```python
from build123d import *

# Parameters (mm, degrees)
BOSS_EXTRUDE1_DEPTH = 58
BOSS_EXTRUDE2_DEPTH = 5
CUT_EXTRUDE1_DEPTH  = 103.78132126
CHAMFER1_SIZE       = 3


with BuildPart() as part:
    # Sketch1 → Boss-Extrude1 (new body)
    with BuildSketch(Plane(origin=(0, 0, 0), x_dir=(1, 0, 0), z_dir=(0, 1, 0))):
        with BuildLine():
            Line((-7, 0), (7, 0))
            ThreePointArc((7, 0), (10.535533906, 1.464466094), (12, 5))
            Line((12, 5), (12, 66.875644347))
            ThreePointArc((12, 66.875644347), (11.829629131, 68.169739573), (11.330127019, 69.375644347))
            Line((11.330127019, 69.375644347), (4.330127019, 81.5))
            ThreePointArc((4.330127019, 81.5), (0, 84), (-4.330127019, 81.5))
            Line((-4.330127019, 81.5), (-11.330127019, 69.375644347))
            ThreePointArc((-11.330127019, 69.375644347), (-11.829629131, 68.169739573), (-12, 66.875644347))
            Line((-12, 66.875644347), (-12, 5))
            ThreePointArc((-12, 5), (-10.535533906, 1.464466094), (-7, 0))
        make_face()
    extrude(amount=BOSS_EXTRUDE1_DEPTH)

    # Sketch2 → Cut-Revolve3 (revolve, cut)
    with BuildSketch(Plane(origin=(0, 0, 0), x_dir=(0, 0, -1), z_dir=(1, 0, 0))):
        Polygon((48, 61), (48, 58), (48, 51.5), (49.5, 50), (48, 48.5), (48, 42), (37.5, 42), (36, 40.5), (34.5, 42), (24, 42), (24, 35.5), (25.5, 34), (24, 32.5), (24, 26), (13.5, 26), (12, 24.5), (10.5, 26), (0, 26), (-2, 26), (-2, 61), align=None)
    revolve(axis=Axis((0, 58, -89), (0, -1, 0)), mode=Mode.SUBTRACT)

    # Sketch3 → Boss-Extrude2 (add)
    with BuildSketch(Plane.XZ):
        with BuildLine():
            Line((-12, -54.599242435), (-12, -57.934874811))
            ThreePointArc((-12, -57.934874811), (0, -55), (12, -57.934874811))
            Line((12, -57.934874811), (12, -54.599242435))
            ThreePointArc((12, -54.599242435), (0, -52), (-12, -54.599242435))
        make_face()
        with BuildLine():
            Line((-12, -62.599242435), (-12, -65.934874811))
            ThreePointArc((-12, -65.934874811), (0, -63), (12, -65.934874811))
            Line((12, -65.934874811), (12, -62.599242435))
            ThreePointArc((12, -62.599242435), (0, -60), (-12, -62.599242435))
        make_face()
        with BuildLine():
            Line((-12, -46.599242435), (-12, -49.934874811))
            ThreePointArc((-12, -49.934874811), (0, -47), (12, -49.934874811))
            Line((12, -49.934874811), (12, -46.599242435))
            ThreePointArc((12, -46.599242435), (0, -44), (-12, -46.599242435))
        make_face()
        with BuildLine():
            Line((-12, -38.599242435), (-12, -41.934874811))
            ThreePointArc((-12, -41.934874811), (0, -39), (12, -41.934874811))
            Line((12, -41.934874811), (12, -38.599242435))
            ThreePointArc((12, -38.599242435), (0, -36), (-12, -38.599242435))
        make_face()
        with BuildLine():
            Line((-12, -30.599242435), (-12, -33.934874811))
            ThreePointArc((-12, -33.934874811), (0, -31), (12, -33.934874811))
            Line((12, -33.934874811), (12, -30.599242435))
            ThreePointArc((12, -30.599242435), (0, -28), (-12, -30.599242435))
        make_face()
        with BuildLine():
            Line((-12, -22.599242435), (-12, -25.934874811))
            ThreePointArc((-12, -25.934874811), (0, -23), (12, -25.934874811))
            Line((12, -25.934874811), (12, -22.599242435))
            ThreePointArc((12, -22.599242435), (0, -20), (-12, -22.599242435))
        make_face()
        with BuildLine():
            Line((-12, -14.599242435), (-12, -17.934874811))
            ThreePointArc((-12, -17.934874811), (0, -15), (12, -17.934874811))
            Line((12, -17.934874811), (12, -14.599242435))
            ThreePointArc((12, -14.599242435), (0, -12), (-12, -14.599242435))
        make_face()
    extrude(amount=BOSS_EXTRUDE2_DEPTH)

    # Sketch4 → Cut-Extrude1 (cut, through all)
    with BuildSketch(Plane.XY):
        with BuildLine():
            Line((12, 16), (8.601411599, 17.071570807))
            ThreePointArc((8.601411599, 17.071570807), (6.817380703, 16.777026114), (6, 15.164136905))
            Line((6, 15.164136905), (6, 8.835863095))
            ThreePointArc((6, 8.835863095), (6.817380703, 7.222973886), (8.601411599, 6.928429193))
            Line((8.601411599, 6.928429193), (12, 8))
            Line((12, 8), (12, 16))
        make_face()
        with BuildLine():
            Line((-12, 8), (-12, 16))
            Line((-12, 16), (-8.601411599, 17.071570807))
            ThreePointArc((-8.601411599, 17.071570807), (-6.817380703, 16.777026114), (-6, 15.164136905))
            Line((-6, 15.164136905), (-6, 8.835863095))
            ThreePointArc((-6, 8.835863095), (-6.817380703, 7.222973886), (-8.601411599, 6.928429193))
            Line((-8.601411599, 6.928429193), (-12, 8))
        make_face()
    extrude(amount=-CUT_EXTRUDE1_DEPTH, mode=Mode.SUBTRACT)

    # Chamfer1
    # the kernel refuses this chamfer: 3.639332034, 3.399408886, 3, 2.719454555, 2.619340105 mm, written as the material it takes off along each edge
    with BuildSketch(Plane(origin=(7, 58, -66.875644347), x_dir=(1, 0, 0), z_dir=(0, 0, 1))) as chamfer1_piece_1:
        Polygon((5 - CHAMFER1_SIZE, 0), (5, -CHAMFER1_SIZE), (5, 0), align=None)
    revolve(axis=Axis((7, 58, -66.875644347), (0, 1, 0)), revolution_arc=30, mode=Mode.SUBTRACT)
    with BuildSketch(Plane(origin=(11.330127019, 58, -69.375644347), x_dir=(0, -1, 0), z_dir=(-0.5000000000000017, 0, -0.8660254037844377)), Plane(origin=(-4.330127019, 58, -81.5), x_dir=(0, -1, 0), z_dir=(-0.5000000000000012, 0, 0.8660254037844379))) as chamfer1_piece_2:
        Polygon((CHAMFER1_SIZE, 0), (0, CHAMFER1_SIZE), (0, 0), align=None)
    extrude(amount=14, mode=Mode.SUBTRACT)
    with BuildSketch(Plane(origin=(0, 58, -79), x_dir=(0.8660254037844403, 0, -0.49999999999999706), z_dir=(0.49999999999999706, 0, 0.8660254037844403))) as chamfer1_piece_3:
        Polygon((5, -CHAMFER1_SIZE), (5 - CHAMFER1_SIZE, 0), (5, 0), align=None)
    revolve(axis=Axis((0, 58, -79), (0, 1, 0)), revolution_arc=120, mode=Mode.SUBTRACT)
    with BuildSketch(Plane(origin=(-7, 58, -66.875644347), x_dir=(-0.866025403784439, 0, -0.4999999999999992), z_dir=(0.4999999999999992, 0, -0.866025403784439))) as chamfer1_piece_4:
        Polygon((5, -CHAMFER1_SIZE), (5 - CHAMFER1_SIZE, 0), (5, 0), align=None)
    revolve(axis=Axis((-7, 58, -66.875644347), (0, 1, 0)), revolution_arc=30, mode=Mode.SUBTRACT)
    with BuildSketch(Plane(origin=(12, 58, -42.080359468), x_dir=(-1, 0, 0), z_dir=(0, 0, -1)), Plane(origin=(-12, 58, -66.875644347), x_dir=(1, 0, 0), z_dir=(0, 0, 1))) as chamfer1_piece_5:
        Polygon((CHAMFER1_SIZE, 0), (0, -CHAMFER1_SIZE), (0, 0), align=None)
    extrude(amount=24.795284879, mode=Mode.SUBTRACT)
    with BuildSketch(Plane(origin=(-12, 42, -43.55256219), x_dir=(0, -1, 0), z_dir=(0, 0, 1)), Plane(origin=(12, 42, -17.402246021), x_dir=(0, -1, 0), z_dir=(0, 0, -1))) as chamfer1_piece_6:
        Polygon((CHAMFER1_SIZE, 0), (0, CHAMFER1_SIZE), (0, 0), align=None)
    extrude(amount=26.150316168, mode=Mode.SUBTRACT)
    with BuildSketch(Plane(origin=(12, 26, 2.715048964), x_dir=(-1, 0, 0), z_dir=(0, 0, -1)), Plane(origin=(-12, 26, -19.13766824), x_dir=(1, 0, 0), z_dir=(0, 0, 1))) as chamfer1_piece_7:
        Polygon((CHAMFER1_SIZE, 0), (0, -CHAMFER1_SIZE), (0, 0), align=None)
    extrude(amount=21.852717204, mode=Mode.SUBTRACT)
    # the kernel refuses this chamfer: 3.639332034, 3.399408886, 3, 2.719454555, 2.619340105 mm, written as the material it takes off along each edge
    with BuildSketch(Plane(origin=(-12, 42, -57.510457396), x_dir=(0, -1, 0), z_dir=(0, 0, 1))) as chamfer1_2_piece_1_section:
        Polygon((CHAMFER1_SIZE, 0), (0, CHAMFER1_SIZE), (0, 0), align=None)
    chamfer1_2_piece_1 = extrude(amount=21.67294417, mode=Mode.PRIVATE)
    chamfer1_2_piece_1 = chamfer1_2_piece_1 - Plane(origin=(0, 42, -89), x_dir=(0, 0, 1), z_dir=(0, -1, 0)) * Cylinder(41, 56, mode=Mode.PRIVATE)
    add(chamfer1_2_piece_1, mode=Mode.SUBTRACT)
    with BuildSketch(Plane(origin=(-12, 26, -32.832343949), x_dir=(0, -1, 0), z_dir=(0, 0, 1))) as chamfer1_2_piece_2_section:
        Polygon((CHAMFER1_SIZE, 0), (0, CHAMFER1_SIZE), (0, 0), align=None)
    chamfer1_2_piece_2 = extrude(amount=21.409724673, mode=Mode.PRIVATE)
    chamfer1_2_piece_2 = chamfer1_2_piece_2 - Plane(origin=(0, 26, -89), x_dir=(0, 0, 1), z_dir=(0, -1, 0)) * Cylinder(65, 55, mode=Mode.PRIVATE)
    add(chamfer1_2_piece_2, mode=Mode.SUBTRACT)
    with BuildSketch(Plane(origin=(12, 26, -11.422619276), x_dir=(0, -1, 0), z_dir=(0, 0, -1))) as chamfer1_2_piece_3_section:
        Polygon((CHAMFER1_SIZE, 0), (0, CHAMFER1_SIZE), (0, 0), align=None)
    chamfer1_2_piece_3 = extrude(amount=21.409724673, mode=Mode.PRIVATE)
    chamfer1_2_piece_3 = chamfer1_2_piece_3 - Plane(origin=(0, 26, -89), x_dir=(0, 0, 1), z_dir=(0, -1, 0)) * Cylinder(65, 55, mode=Mode.PRIVATE)
    add(chamfer1_2_piece_3, mode=Mode.SUBTRACT)
    with BuildSketch(Plane(origin=(12, 42, -35.837513226), x_dir=(0, -1, 0), z_dir=(0, 0, -1))) as chamfer1_2_piece_4_section:
        Polygon((CHAMFER1_SIZE, 0), (0, CHAMFER1_SIZE), (0, 0), align=None)
    chamfer1_2_piece_4 = extrude(amount=21.67294417, mode=Mode.PRIVATE)
    chamfer1_2_piece_4 = chamfer1_2_piece_4 - Plane(origin=(0, 42, -89), x_dir=(0, 0, 1), z_dir=(0, -1, 0)) * Cylinder(41, 56, mode=Mode.PRIVATE)
    add(chamfer1_2_piece_4, mode=Mode.SUBTRACT)


solid = part.part
```
Build history of the part. All positions in model axes, mm. A direction names the side the tool comes from. Coordinates: 2 decimals unless noted, no trailing zeros. Order: outer loops, then holes, each group sorted by start corner. A loop starts at its lowest first (then second) coordinate and runs counter-clockwise, first axis right, second up. Notation, with made-up numbers: (26.5, -30.5) -> (30.5, -30.5) arc R11 cw to (30.5, -16.5) -> close; hole circle Ø9 at (75, -10). An arc over 180 degrees is marked (long way). Answer in a Markdown table with one row per item. Add a question column.
Q1. Drop flat-ended pins along their axis: pin 1 (8 mm diameter, centred on x = -3, y = 29, fed in from +Z); pin 2 (2 mm diameter, centred on x = -3.5, y = 46.5, fed in from -Z); pin 3 (5.5 mm diameter, centred on x = -2, z = -20, fed in from +Y); pin 4 (3.5 mm diameter, centred on x = -2, z = -29.5, fed in from +Y). Give the stop position or say it passes through.
Q2. Wall check: line 1 along X through (y, z) = (10, -68); line 2 along Y through (x, z) = (3, -68); line 3 along Y through (x, z) = (2.5, -23.5). Give the ranges that are in metal, low to high. Write a range as [from, to].
Q3. Band-saw the part on A-A, the plane y = 29.5. List the corners of the cut face in (x, z), then the cut area to 3 significant figures.
Q4. Band-saw the part on B-B, the plane z = -6. List the corners of the cut face in (x, y).
Q5. Band-saw the part on C-C, the plane y = 3.5. List the corners of the cut face in (x, z).
Q6. Mould opens along Z. For faces 6 (the face through (10, 4, -1)), 7 (the face through (0, -2, -23)), 8 (the face through (-10, 57, -58)) say: +Z half, -Z half, draft (parallel to the pull), parting line (faces both ways), or undercut.
Q7. Which spindle directions (+Z, -Z, +X, -X, +Y, -Y) get a long thin tool onto all of the face, cutting with end or side? Do faces 1 (the face through (-11.825, 3.944, -68.187)), 2 (the face through (-6.839, 16.792, -38.754)), 3 (the face through (0, -2, -36)), 4 (the face through (0.2, 49.6, -49.1)), 5 (the face through (0, -2, -12)). Say none if no direction does.
Q8. Band-saw the part on D-D, the plane z = -75. List the corners of the cut face in (x, y), then the cut area to 3 significant figures.
Answers follow:
| question | item | result |
|---|---|---|
| 1 | pin 1 | z = 0 |
| 1 | pin 2 | z = -83.33 |
| 1 | pin 3 | y = 26 |
| 1 | pin 4 | y = 42 |
| 2 | line 1 | [-6, 6] |
| 2 | line 2 | [0, 58] |
| 2 | line 3 | [0, 26] |
| 3 | outline | (-12, -66.88) arc R5 ccw to (-11.33, -69.38) -> (-4.33, -81.5) arc R5 ccw to (4.33, -81.5) -> (11.33, -69.38) arc R5 ccw to (12, -66.88) -> (12, -25.12) arc R65 ccw to (-12, -25.12) -> close |
| 3 | area | 1,280 mm^2 |
| 4 | outline | (-12, 0) -> (12, 0) -> (12, 8) -> (8.6, 6.93) arc R2 cw to (6, 8.84) -> (6, 15.16) arc R2 cw to (8.6, 17.07) -> (12, 16) -> (12, 23) -> (9, 26) -> (-9, 26) -> (-12, 23) -> (-12, 16) -> (-8.6, 17.07) arc R2 cw to (-6, 15.16) -> (-6, 8.84) arc R2 cw to (-8.6, 6.93) -> (-12, 8) -> close |
| 5 | outline | (-12, -66.88) arc R5 ccw to (-11.33, -69.38) -> (-4.33, -81.5) arc R5 ccw to (4.33, -81.5) -> (11.33, -69.38) arc R5 ccw to (12, -66.88) -> (12, -5) arc R5 ccw to (7, 0) -> (-7, 0) arc R5 ccw to (-12, -5) -> close |
| 6 | face 6 | +Z half |
| 6 | face 7 | undercut |
| 6 | face 8 | draft |
| 7 | face 1 | -Z, -X, +Y, -Y |
| 7 | face 2 | +Z, -Z |
| 7 | face 3 | -Y |
| 7 | face 4 | +Z |
| 7 | face 5 | +Z, -Y |
| 8 | outline | (-8.08, 0) -> (8.08, 0) -> (8.08, 6.84) arc R2 cw to (6, 8.84) -> (6, 15.16) arc R2 cw to (8.08, 17.16) -> (8.08, 55) -> (4.62, 58) -> (-4.62, 58) -> (-8.08, 55) -> (-8.08, 17.16) arc R2 cw to (-6, 15.16) -> (-6, 8.84) arc R2 cw to (-8.08, 6.84) -> close |
| 8 | area | 888 mm^2 |
